Geometry: see drawing. Coordinates: mm, zero at the bounding-box minimum. Coordinates: 2 decimals unless noted, no trailing zeros. Order: outer loops, then holes, each group sorted by start corner. A loop starts at its lowest first (then second) coordinate and runs counter-clockwise, first axis right, second up.
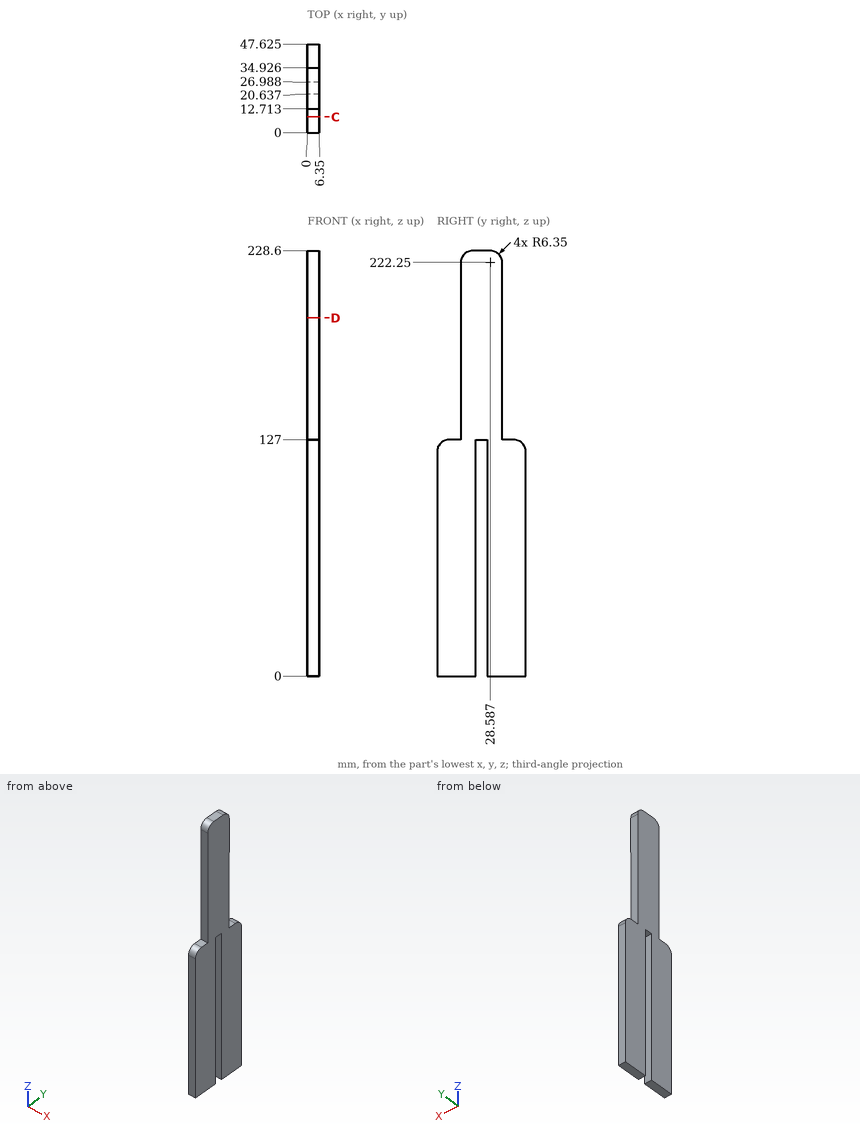
Q1. Pin query (flat end, axial travel): P1, Ø1.9, axis at x = 4, z = 179.5, coming from the +Y side; P2, Ø3, axis at x = 3.5, y = 24.5, coming from the -Z side; P3, Ø1.9, axis at x = 3.5, y = 10.5, coming from the +Z side. Return the tip coordinate at first contact, or that it passes through.
Solutions:
P1: stops at y = 34.93
P2: stops at z = 127
P3: stops at z = 127
Q2. Material intervals for line 1 along Y through (x, z) = (3.75, 46) (1 decimal); line 2 along Z through (x, y) = (3.25, 10); line 3 along Y through (x, z) = (2.5, 202) (1 decimal), sorted ascending.
Solutions:
line 1: y = 0 to 20.6, 27 to 47.6
line 2: z = 0 to 127
line 3: y = 12.7 to 34.9
Q3. Section query D-D on z = 192.5. Output: boundary loops of the cut face in (x, y), plus the area to 3 significant figures.
Solutions:
outline: (0, 12.71) - (6.35, 12.71) - (6.35, 34.93) - (0, 34.93) - close
area: 141 mm2
Q4. Section query C-C on y = 8.5. Output: boundary loops of the cut face in (x, z).
Solutions:
outline: (0, 0) - (6.35, 0) - (6.35, 127) - (0, 127) - close
